```python
from build123d import *

# Parameters (mm, degrees)
SKETCH1_W                       = 10.16
SKETCH1_H                       = 3.175
BOSS_EXTRUDE1_DEPTH             = 4.445
SKETCH3_OUTSIDE_W               = 14.934
SKETCH3_OUTSIDE_H               = 13.664
SKETCH3_OUTSIDE_W_2             = 10.16
SKETCH3_OUTSIDE_H_2             = 8.89
SKETCH3_OUTSIDE_W_3             = 5.08
SKETCH3_OUTSIDE_H_3             = 5.08
CUT_EXTRUDE1_DEPTH              = 1.905
BOSS_EXTRUDE2_REACH             = 6.445
BOSS_EXTRUDE2_DIRECTION_2_REACH = 6.445
CUT_EXTRUDE3_DEPTH              = 5.445
CUT_EXTRUDE3_DEPTH_BACK         = 5.445


with BuildPart() as part:
    # Sketch1 → Boss-Extrude1 (new body, symmetric)
    with BuildSketch(Plane.XY):
        with Locations((0, -1.5875)):
            Rectangle(SKETCH1_W, SKETCH1_H)
    extrude(amount=BOSS_EXTRUDE1_DEPTH, both=True)

    # Sketch3 outside → Cut-Extrude1 (cut)
    with BuildSketch(Plane.XZ.offset(3.175)):
        Rectangle(SKETCH3_OUTSIDE_W, SKETCH3_OUTSIDE_H)
        Rectangle(SKETCH3_OUTSIDE_W_2, SKETCH3_OUTSIDE_H_2, mode=Mode.SUBTRACT)
        Rectangle(SKETCH3_OUTSIDE_W_3, SKETCH3_OUTSIDE_H_3)
    extrude(amount=-CUT_EXTRUDE1_DEPTH, mode=Mode.SUBTRACT)

    # Boss-Extrude2: up to this face of the body (flat: up to its plane)
    boss_extrude2_end = Plane(part.part.faces().sort_by_distance((0, -1.5875, 4.445))[0])
    # Sketch5 → Boss-Extrude2 (add, up to the picked face)
    with BuildSketch(Plane.XY, mode=Mode.PRIVATE) as boss_extrude2_sk1:
        Polygon((-2.924444558, 0), (5.08, 3.81), (5.08, 0), align=None)
    boss_extrude2_tool1 = split(extrude(boss_extrude2_sk1.sketch, amount=BOSS_EXTRUDE2_REACH, mode=Mode.PRIVATE), bisect_by=boss_extrude2_end, keep=Keep.BOTH, mode=Mode.PRIVATE)
    add(boss_extrude2_tool1.solids().sort_by_distance((2.411852, 1.27, 0))[0])

    # Boss-Extrude2 direction 2: up to this face of the body (flat: up to its plane)
    boss_extrude2_direction_2_end = Plane(part.part.faces().sort_by_distance((0, -1.5875, -4.445))[0])
    # Sketch5 → Boss-Extrude2 direction 2 (add, up to the picked face)
    with BuildSketch(Plane.XY, mode=Mode.PRIVATE) as boss_extrude2_direction_2_sk1:
        Polygon((-2.924444558, 0), (5.08, 3.81), (5.08, 0), align=None)
    boss_extrude2_direction_2_tool1 = split(extrude(boss_extrude2_direction_2_sk1.sketch, amount=-BOSS_EXTRUDE2_DIRECTION_2_REACH, mode=Mode.PRIVATE), bisect_by=boss_extrude2_direction_2_end, keep=Keep.BOTH, mode=Mode.PRIVATE)
    add(boss_extrude2_direction_2_tool1.solids().sort_by_distance((2.411852, 1.27, 0))[0])

    # Sketch6 → Cut-Extrude3 (cut, two sides)
    with BuildSketch(Plane.XY) as cut_extrude3_sk:
        Polygon((-5.08, -1.026013257), (-5.08, 0), (-2.924444558, 0), align=None)
    extrude(amount=CUT_EXTRUDE3_DEPTH, mode=Mode.SUBTRACT)
    extrude(cut_extrude3_sk.sketch, amount=-CUT_EXTRUDE3_DEPTH_BACK, mode=Mode.SUBTRACT)


solid = part.part
```
Model file for the job. Use its own axes, mm. A direction names the side the tool comes from. Round coordinates to 2 decimals unless told otherwise and drop trailing zeros. Write each loop counter-clockwise with the first axis right and the second up, starting at its lowest first coordinate (ties: lowest second). Pieces come first, ordered by that corner, then holes. Notation, with made-up numbers: (46.25, -6) - (98.25, -6) arc R10 cw to (98.25, 6) - close; hole circle Ø10 at (4, 60). An arc over 180 degrees is marked (long way). One line per item, written item: value.
(1) Cut at A-A, the plane y = -1.5. Give the cut face in (x, z) (3 decimals).
Values follow:
outline: (-5.08, -4.445) - (5.08, -4.445) - (5.08, 4.445) - (-5.08, 4.445) - close; hole (-2.54, -2.54) - (2.54, -2.54) - (2.54, 2.54) - (-2.54, 2.54) - close
(2) Cut at D-D, the plane y = 1.5. Give the cut face in (x, z) (3 decimals).
Values follow:
outline: (0.227, -4.445) - (5.08, -4.445) - (5.08, 4.445) - (0.227, 4.445) - close
(3) Two-plate mould, pull along X, no slides. Class faces 3 (the flat face through (-5.08, -2, 0)), 4 (the flat face through (2.54, -2, 0)), 5 (the flat face through (1, 0, 4.445)): pulls with the +X half, pulls with the -X half, needs draft (parallel to the pull), parting line crosses it, or undercut.
Values follow:
face 3: pulls with the -X half
face 4: undercut
face 5: needs draft
(4) Wall check: probe 1 along Z at (x, y) = (-1.5, -2) (3 decimals); probe 2 along X at (y, z) = (-1.75, -2.25); probe 3 along X at (y, z) = (-0.75, -3.5). Give the ranges that are in metal, low to high.
Values follow:
probe 1: z = -4.445 to -2.54, 2.54 to 4.445
probe 2: x = -5.08 to -2.54, 2.54 to 5.08
probe 3: x = -4.5 to 5.08
(5) Cut at C-C, the plane x = 0.5. Give the cut face in (y, z) (3 decimals).
Values follow:
outline: (-3.175, -4.445) - (1.63, -4.445) - (1.63, 4.445) - (-3.175, 4.445) - (-3.175, 2.54) - (-1.27, 2.54) - (-1.27, -2.54) - (-3.175, -2.54) - close
(6) Cut at B-B, the plane z = -2.75. Give the cut face in (x, y) (3 decimals).
Values follow:
outline: (-5.08, -3.175) - (5.08, -3.175) - (5.08, 3.81) - (-5.08, -1.026) - close
(7) 3-axis set-ups, long thin cutter, end or side, ignore diameter. For faces 1 (the flat face through (0, -3.175, 3)), 2 (the flat face through (-2.54, -2, 0)): which of +Z, -Z, +X, -X, +Y, -Y reach the whole face in a straight line?
Values follow:
face 1: +Z, -Z, +X, -X, -Y
face 2: -Y
(8) Drop flat-ended pins along their axis: P1, Ø1.5, axis at x = 4, z = -2.5, coming from the +Y side; P2, Ø1, axis at x = -3.5, z = 2, coming from the +Y side; P3, Ø3, axis at x = 3, z = -2.5, coming from the +Y side. Give the stop position or say it passes through.
Values follow:
P1: stops at y = 3.65
P2: stops at y = -0.04
P3: stops at y = 3.53
